Could you check a few things on this model? Use its own coordinates, in mm. A direction names the side the tool comes from. Coordinates: 2 decimals unless noted, no trailing zeros. Order: outer loops, then holes, each group sorted by start corner. A loop starts at its lowest first (then second) coordinate and runs counter-clockwise, first axis right, second up. Notation, with made-up numbers: (-6, -19) -> (24, -19) arc R26 ccw to (24, 13) -> close; hole circle Ø7 at (72.5, 56). An arc over 180 degrees is marked (long way). Use a Markdown table: item, result. Add a question column.
1) If we section it at B-B (y = 0): Write out the boundary of the cut face in (x, z).
2) If I drill on L1, parallel to Y at x = 8, z = 0.8; L2, parallel to X at y = -1.25, z = 2.5; L3, parallel to X at y = 0, z = 0.75, over which ranges is the centre line in solid material (lowest first)? Write a range as [from, to].
3) Which directions (+Z, -Z, +X, -X, +Y, -Y) give clear straight access to the entire face, cutting with the end or side of a thin tool? Please do faces 1 (the flat face through (8, 14, 2)), 2 (the cylindrical face through (7.5, -4.22, 1.8)), 3 (the flat face through (15.5, 0, 1)).
4) Thinking about a two-plate mould opening in X: for faces 4 (the flat face through (14.8, -0.2, 2.7)), 5 (the flat face through (7, -8, 1.6)), 6 (the flat face through (6, -15, 1)), which applies, +X half, -X half, draft (parallel to the pull), parting line (faces both ways), or undercut?
5) If we section it at D-D (x = 1.5): Write out the boundary of the cut face in (y, z).
6) If we section it at C-C (z = 1): Write out the boundary of the cut face in (x, y).
7) Will these pins go through, and if not, where does the flat tip stop? pin 1 Ø0.6 at (x, y) = (6.5, -14) entering from +Z; pin 2 Ø2 at (x, y) = (12.5, -1.5) entering from +Z; pin 3 Ø5 at (x, y) = (8, 0) entering from -Z.
8) If we section it at A-A (x = 8): Write out the boundary of the cut face in (y, z), plus the area to 3 significant figures.
```python
from build123d import *

# Parameters (mm, degrees)
PAD_DEPTH       = 15
SKETCH001_R     = 2.25
HOLE_DEPTH      = 6.001
POCKET010_DEPTH = 0.4
CHAMFER004_SIZE = 0.4


with BuildPart() as part:
    # Sketch → Pad (new body, symmetric)
    with BuildSketch(Plane.XZ):
        Polygon((0, 6), (0, 0), (15.5, 0), (15.5, 2), (14, 3.5), (12.5, 2), (2.5, 2), (2.5, 3.5), align=None)
    extrude(amount=PAD_DEPTH, both=True)

    # Sketch001 → Hole (cut, through all)
    with BuildSketch(Plane.XY):
        with Locations((8, 0)):
            Circle(SKETCH001_R)
    extrude(amount=HOLE_DEPTH, mode=Mode.SUBTRACT)

    # Sketch013 (on Face11 of Hole) → Pocket010 (cut)
    with BuildSketch(Plane(origin=(0, 0, 2), x_dir=(-1, 0, 0), z_dir=(0, 0, 1))):
        with BuildLine():
            Line((-12.5, 13), (-2.5, 13))
            Line((-2.5, 13), (-2.5, 1.2))
            Line((-2.5, 1.2), (-3.92293, 1.2))
            ThreePointArc((-3.92293, 1.2), (-7.565024, 4.227682), (-11.747312, 2.005032))
            ThreePointArc((-12.5, 2.193741), (-12.197275, 1.805749), (-11.747312, 2.005032))
            Line((-12.5, 2.193741), (-12.5, 13))
        make_face()
        with BuildLine():
            Line((-12.5, -13), (-2.5, -13))
            Line((-2.5, -13), (-2.5, -1.2))
            Line((-2.5, -1.2), (-3.92293, -1.2))
            ThreePointArc((-11.747312, -2.005032), (-7.565024, -4.227682), (-3.92293, -1.2))
            ThreePointArc((-11.747312, -2.005032), (-12.197275, -1.805749), (-12.5, -2.193741))
            Line((-12.5, -2.193741), (-12.5, -13))
        make_face()
    extrude(amount=-POCKET010_DEPTH, mode=Mode.SUBTRACT)

    # Chamfer004
    chamfer004_edges = [part.edges().sort_by_distance(p)[0] for p in [
        (0, 0, 0),
        (7.75, 15, 0),
        (7.75, -15, 0),
        (15.5, 0, 0),
        (10.25, 0, 0),
    ]]
    chamfer(chamfer004_edges, length=CHAMFER004_SIZE)


solid = part.part
```
Answer sheet:
| question | item | result |
|---|---|---|
| 1 | outline | (0, 0.4) -> (0.4, 0) -> (5.35, 0) -> (5.75, 0.4) -> (5.75, 2) -> (2.5, 2) -> (2.5, 3.5) -> (0, 6) -> close; (10.25, 0.4) -> (10.65, 0) -> (15.1, 0) -> (15.5, 0.4) -> (15.5, 2) -> (14, 3.5) -> (12.5, 2) -> (10.25, 2) -> close |
| 2 | L1 | [-15, -2.25], [2.25, 15] |
| 2 | L2 | [0, 2.5], [13, 15] |
| 2 | L3 | [0, 5.75], [10.25, 15.5] |
| 3 | face 1 | +Z, +Y, -Y |
| 3 | face 2 | +Z |
| 3 | face 3 | +Z, -Z, +X, +Y, -Y |
| 4 | face 4 | +X half |
| 4 | face 5 | undercut |
| 4 | face 6 | draft |
| 5 | outline | (-15, 0.4) -> (-14.6, 0) -> (14.6, 0) -> (15, 0.4) -> (15, 4.5) -> (-15, 4.5) -> close |
| 6 | outline | (0, -15) -> (15.5, -15) -> (15.5, 15) -> (0, 15) -> close; hole circle Ø4.5 at (8, 0) |
| 7 | pin 1 | z = 2 |
| 7 | pin 2 | z = 3 |
| 7 | pin 3 | z = 0.15 |
| 8 | outline | (-15, 0.4) -> (-14.6, 0) -> (-2.65, 0) -> (-2.25, 0.4) -> (-2.25, 2) -> (-4.25, 2) -> (-4.25, 1.6) -> (-13, 1.6) -> (-13, 2) -> (-15, 2) -> close; (2.25, 0.4) -> (2.65, 0) -> (14.6, 0) -> (15, 0.4) -> (15, 2) -> (13, 2) -> (13, 1.6) -> (4.25, 1.6) -> (4.25, 2) -> (2.25, 2) -> close |
| 8 | area | 43.7 mm2 |
